Could you check a few things on this drawing? It's one solid part, dimensions in mm from its lowest x, y, z. Round coordinates to 2 decimals unless told otherwise and drop trailing zeros. Order: outer loops, then holes, each group sorted by start corner. A loop starts at its lowest first (then second) coordinate and runs counter-clockwise, first axis right, second up.
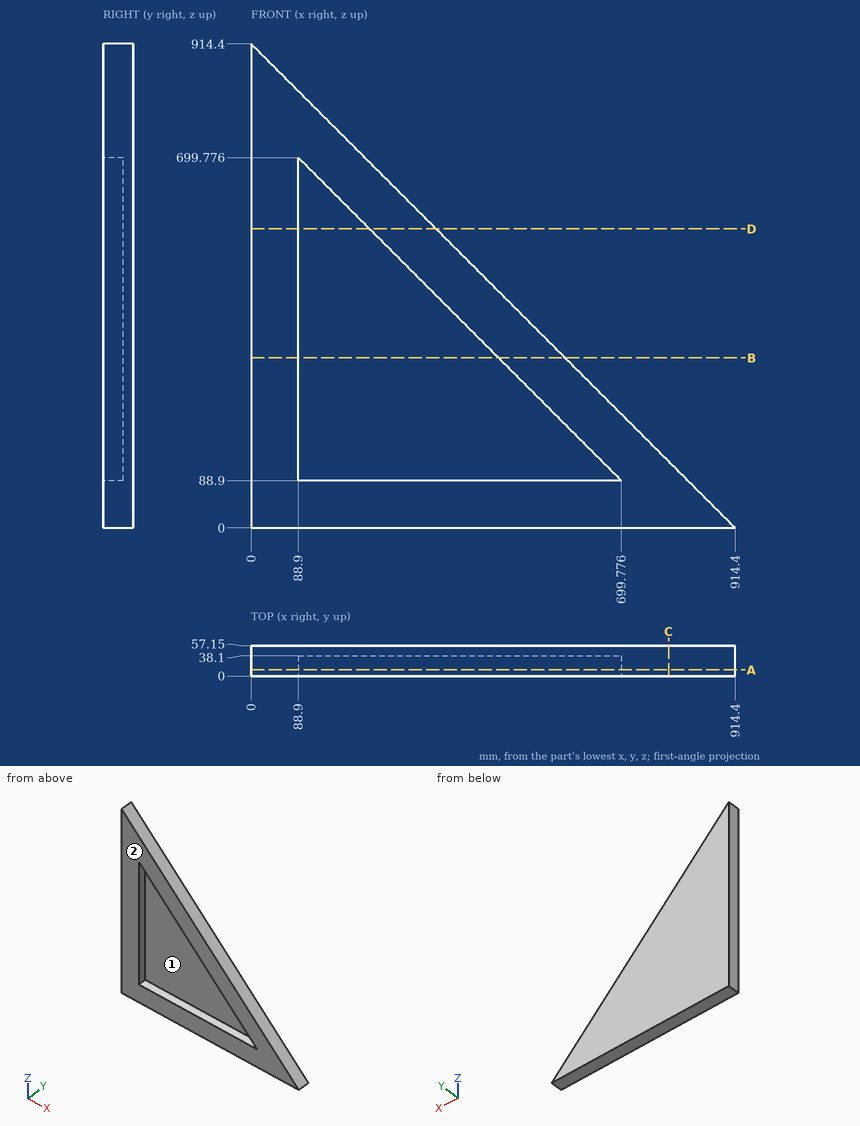
1) I'm going to push flat-ended pins straight in: pin 1 (1 mm diameter, centred on y = 31, z = 503, fed in from +X); pin 2 (19 mm diameter, centred on x = 313, y = 10, fed in from +Z); pin 3 (1.5 mm diameter, centred on x = 207, z = 189, fed in from -Y). Where does each tip first touch, or does it pass through?
2) If we section it at B-B (z = 321): Write out the boundary of the cut face in (x, y), plus the area to 3 significant figures.
3) We'd pull the mould along X, two halves only. Please class the marked faces 1 and 2: +X half, -X half, draft (parallel to the pull), parting line (faces both ways), or undercut.
4) If we section it at C-C (x = 789): Write out the boundary of the cut face in (y, z), plus the area to 3 significant figures.
5) I need wall thicknesses on line 1 (Y direction, x = 509, z = 106); line 2 (X direction, y = 18, z = 246) (1 decimal); line 3 (Z direction, x = 610.5, y = 28.5) (1 decimal). Which ranges of each line are inside material? Lowest first, please.
6) If we section it at D-D (z = 565): Write out the boundary of the cut face in (x, y), plus the area to 3 significant figures.
7) If we section it at A-A (y = 11.5): Write out the boundary of the cut face in (x, z).
Solutions:
1. pin 1: stops at x = 411.9
1. pin 2: stops at z = 610.9
1. pin 3: stops at y = 38.1
2. outline: (0, 0) - (88.9, 0) - (88.9, 38.1) - (467.68, 38.1) - (467.68, 0) - (593.4, 0) - (593.4, 57.15) - (0, 57.15) - close
2. area: 19,500 mm2
3. face 1: undercut
3. face 2: draft
4. outline: (0, 0) - (57.15, 0) - (57.15, 125.4) - (0, 125.4) - close
4. area: 7,170 mm2
5. line 1: y = 38.1 to 57.15
5. line 2: x = 0 to 88.9, 542.7 to 668.4
5. line 3: z = 0 to 88.9, 178.2 to 303.9
6. outline: (0, 0) - (88.9, 0) - (88.9, 38.1) - (223.68, 38.1) - (223.68, 0) - (349.4, 0) - (349.4, 57.15) - (0, 57.15) - close
6. area: 14,800 mm2
7. outline: (0, 0) - (914.4, 0) - (0, 914.4) - close; hole (88.9, 88.9) - (699.78, 88.9) - (88.9, 699.78) - close
